Input: part model. Units: mm. Frame: model coordinates. A direction names the side the tool comes from. Give positions to 0.01 mm unless a question says otherwise; leave off trailing zeros. Loops run counter-clockwise (first coordinate to the right, second up) from the corner with the lowest first, then second, coordinate; pieces in that order, holes last. Notation, with made-up numbers: M -36.5,-28 L 18.5,-28 A27 cw 18.5,-11 Z; hole C -28,83 d8. An arc over 180 degrees is marked long. Answer as a JSON object with one key per item and string values. Group by question number.
1) First-contact query: P1, Ø8, axis at x = -43.5, y = 197.5, coming from the +Z side; P2, Ø2, axis at x = -62, z = -93.5, coming from the -Y side; P3, Ø6, axis at x = -29.5, y = 15.5, coming from the +Z side. Flat tips, straight axial feed; report the tip coordinate or a pass-through.
2) Access query for faces 5 (the flat face through (100, -1, -168)), 6 (the flat face through (-1, 75, -51)), 7 (the cylindrical face through (-47.69, -15.02, -267.35)). Directions: +Z, -Z, +X, -X, +Y, -Y. A direction counts if a zero-diameter tool reaches every point of the face in a straight line with its end or side. Return the directions, or none.
3) Section query A-A on x = 0. Return loops of the section in (y, z).
4) Section query C-C on y = 0. Return loops of the section in (x, z).
5) Section query B-B on z = -42.5. Return loops of the section in (x, y).
6) Ray query, L1, parallel to Z at x = 0, y = 87; L2, parallel to X at y = 82, z = 0; L3, parallel to Y at x = -69.5, z = -169.5. Return the intervals inside material, ascending.
7) Draft query along X for faces 1 (the flat face through (1, -100, -81)), 2 (the cylindrical face through (249.76, -10.99, -361.25)), 3 (the cylindrical face through (-47.69, -87.32, 15.02)), 4 (the flat face through (-100, -1, -165)). Return one class per face: +X half, -X half, draft (parallel to the pull), parting line (faces both ways), or undercut.
8) Section query D-D on y = 61. Return loops of the section in (x, z), plus the area to 3 significant figures.
Autodesk Inventor part; units mm, degrees
ref_plane "YZ Plane" through (0, 0, 0) normal (1, 0, 0) x (0, 1, 0)
ref_plane "XZ Plane" through (0, 0, 0) normal (0, 1, 0) x (-1, 0, 0)
ref_plane "XY Plane" through (0, 0, 0) normal (0, 0, 1) x (1, 0, 0)
sketch "Sketch2" plane through (0, 0, 0) normal (0, 1, 0) x (-1, 0, 0)
  line L0 (0, 143.7774) -> (0, -86.6025) construction
  line L1 (190.8875, 0) -> (-168.3726, 0)
  arc A0 (50, -86.6025) -> (0, 100) centre (0, 0) ccw construction
  line L2 (0, 0) -> (0, -86.6025) construction
  line L3 (0, -386.6025) -> (250, -386.6025)
  line L4 (250, -386.6025) -> (250, -336.6025)
  line L5 (250, -336.6025) -> (50, -336.6025)
  line L6 (50, -336.6025) -> (50, -86.6025)
  line L7 (0, 0) -> (0, 100) construction
  line L8 (50, -86.6025) -> (0, -86.6025)
  line L9 (0, -86.6025) -> (0, -95.5661) construction
  line L10 (0, -86.6025) -> (0, -386.6025)
  dimension "d0" = 100
  dimension "ht" = 250
  dimension "base_thick" = 50
  dimension "base_radius" = 250
  dimension "d11" = 50
revolve "Revolution2" add sketch "Sketch2" angle 360 about axis through (0, 0, 143.7774) along (0, 0, -1)
sketch "Sketch3" plane through (0, 0, 0) normal (0, 1, 0) x (-1, 0, 0)
  line L0 (68.3369, 0) -> (-71.9882, 0)
  line L1 (0, 52.8788) -> (0, -69.4874)
  arc A0 (100, 0) -> (-100, 0) centre (0, 0) ccw
  line L2 (100, 0) -> (100, -200)
  line L3 (100, -200) -> (-100, -200)
  line L4 (-100, -200) -> (-100, 0)
  dimension "d26" = 100
  dimension "d27" = 200
extrude "Extrusion1" add sketch "Sketch3" along normal mid plane 200
sketch "Sketch4" plane through (0, 0, 0) normal (0, 1, 0) x (-1, 0, 0)
  circle A0 centre (0, 0) radius 50
  dimension "d30" = 50
extrude "Extrusion2" cut sketch "Sketch4" along normal through all both and the other way through all
sketch "Sketch5" plane through (0, 0, 0) normal (1, 0, 0) x (0, 1, 0)
  line L0 (75, -150) -> (-75, -150)
  line L1 (-75, -150) -> (-75, 100)
  line L2 (-75, 100) -> (75, 100)
  line L3 (75, 100) -> (75, -150)
  line L4 (0, -62.7821) -> (0, 60)
  line L5 (91.6333, 0) -> (-95.5004, 0)
  line L6 (0, -400) -> (0, 300) construction
  point P0 (0, 0)
  dimension "d35" = 75
  dimension "d36" = 100
  dimension "d39" = 150
extrude "Extrusion3" cut sketch "Sketch5" along normal through all both and the other way through all
equation "\"d0\" = S_radius"
equation "\"ht\" = 5 * rod_radius"
equation "\"base_thick\" = rod_radius"
equation "\"base_radius\" = 5 * rod_radius"
equation "\"d11\" = rod_radius"
equation "\"d26\" = S_radius"
equation "\"d27\" = 2 * S_radius"
equation "\"d28\" = 2 * S_radius"
equation "\"d30\" = rod_radius"
equation "\"d35\" = 1.5 * rod_radius"
equation "\"d36\" = S_radius"
equation "\"d39\" = 1.5 * S_radius"
equation "\"rod_radius\" = 50"
equation "\"S_radius\" = 2 * rod_radius"
properties part number "FP"
Output:
{
 "1": {"P1": "stops at z = -336.6", "P2": "stops at y = -100", "P3": "stops at z = -150"},
 "2": {"face 5": "+Z, +X, +Y, -Y", "face 6": "+Z, +X, -X", "face 7": "none"},
 "3": {"outline": "M -250,-386.6 L 250,-386.6 L 250,-336.6 L 50,-336.6 L 50,-200 L 100,-200 L 100,-50 L 75,-50 L 75,-150 L -75,-150 L -75,-50 L -100,-50 L -100,-200 L -50,-200 L -50,-336.6 L -250,-336.6 Z; M -100,50 L -75,50 L -75,100 L -100,100 Z; M 75,50 L 100,50 L 100,100 L 75,100 Z"},
 "4": {"outline": "M -250,-386.6 L 250,-386.6 L 250,-336.6 L 50,-336.6 L 50,-200 L 100,-200 L 100,-150 L -100,-150 L -100,-200 L -50,-200 L -50,-336.6 L -250,-336.6 Z"},
 "5": {"outline": "M -100,-100 L -26.34,-100 L -26.34,-75 L -100,-75 Z; M -100,75 L -26.34,75 L -26.34,100 L -100,100 Z; M 26.34,-100 L 100,-100 L 100,-75 L 26.34,-75 Z; M 26.34,75 L 100,75 L 100,100 L 26.34,100 Z"},
 "6": {"L1": "z = -386.6 to -336.6, -200 to -50, 50 to 100", "L2": "x = -100 to -50, 50 to 100", "L3": "y = -100 to 100"},
 "7": {"face 1": "draft", "face 2": "parting line", "face 3": "undercut", "face 4": "-X half"},
 "8": {"outline": "M -242.44,-386.6 L 242.44,-386.6 L 242.44,-336.6 L -242.44,-336.6 Z; M -100,-200 L 100,-200 L 100,-150 L -100,-150 Z", "area": "34,200 mm^2"}
}
